```python
from build123d import *

# Parameters (mm, degrees)
F0_W     = 55
F0_H     = 62
F0_W_2   = 7.5
F1_DEPTH = 16.7
F2_T     = -2


with BuildPart() as f1:
    # F0 (on Top) → F1 (new body)
    with BuildSketch(Plane.XY):
        with Locations((27.5, 31)):
            Rectangle(F0_W, F0_H)
        with Locations((-3.75, 31)):
            Rectangle(F0_W_2, F0_H)
    extrude(amount=-F1_DEPTH)

    # F2
    f2_openings = [f1.faces().sort_by_distance(p)[0] for p in [
        (-7.5, 31, -8.35),
    ]]
    offset(amount=F2_T, openings=f2_openings)


solid = f1.part
```
Source: CAD feature listing. Evaluate the final solid. Frame: model axes, mm. A direction names the side the tool comes from. Round coordinates to 2 decimals unless told otherwise and drop trailing zeros. Loops run counter-clockwise (first coordinate to the right, second up) from the corner with the lowest first, then second, coordinate; pieces in that order, holes last.
1. Mould query, pull axis Z, two halves, no side actions, for faces 3 (the flat face through (23, 0, -8)), 4 (the flat face through (22, 31, -2)), 5 (the flat face through (23, 31, -16.7)). Classes: released by +Z, released by -Z, zero draft, split by the parting line, or undercut.
2. Section query B-B on z = -13.25. Output: boundary loops of the cut face in (x, y), and give its area (3 significant figures).
3. Section query A-A on x = 3.5. Output: boundary loops of the cut face in (y, z).
4. Contact query for flat-ended pins moving along their axis: pin 1 (6 mm diameter, centred on x = 2, z = -4, fed in from -Y); pin 2 (6.5 mm diameter, centred on y = 28, z = -11, fed in from -X). Output: stop coordinate, or through.
5. Access query for faces 1 (the flat face through (53, 31, -8)), 2 (the flat face through (-7.5, 29, -15)). Directions: +Z, -Z, +X, -X, +Y, -Y. A direction counts if a zero-diameter tool reaches every point of the face in a straight line with its end or side. Return the directions, or none.
6. Ray query, L1, parallel to Y at x = 44, z = -4.25; L2, parallel to Z at x = 25, y = 8; L3, parallel to X at y = 28.5, z = -7.5. Return the intervals inside material, ascending.
7. Section query C-C on y = 51.5. Output: boundary loops of the cut face in (x, z), and give its area (3 significant figures).
Answers below:
1. face 3: zero draft
1. face 4: undercut
1. face 5: released by -Z
2. outline: (-7.5, 0) - (55, 0) - (55, 62) - (-7.5, 62) - (-7.5, 60) - (53, 60) - (53, 2) - (-7.5, 2) - close
2. area: 366 mm2
3. outline: (0, -16.7) - (62, -16.7) - (62, 0) - (0, 0) - close; hole (2, -14.7) - (60, -14.7) - (60, -2) - (2, -2) - close
4. pin 1: stops at y = 0
4. pin 2: stops at x = 53
5. face 1: -X
5. face 2: +Z, -Z, -X, +Y, -Y
6. L1: y = 0 to 2, 60 to 62
6. L2: z = -16.7 to -14.7, -2 to 0
6. L3: x = 53 to 55
7. outline: (-7.5, -16.7) - (55, -16.7) - (55, 0) - (-7.5, 0) - (-7.5, -2) - (53, -2) - (53, -14.7) - (-7.5, -14.7) - close
7. area: 275 mm2
